Answer from the drawing. Dimensions are ordinates in mm from the lowest x, y and z of the part. Coordinates: 2 decimals unless noted, no trailing zeros. Loops run counter-clockwise (first coordinate to the right, second up) from the corner with the lowest first, then second, coordinate; pieces in that order, holes last. Notation, with made-up numbers: (-2.5, 9.25) - (51.5, 9.25) arc R14 ccw to (51.5, 15.25) - close; hole circle Ø7 at (43.25, 18). An arc over 180 degrees is marked (long way). Write each question's results on one line, items separated by ' | '. Start each with the question number.
1. Find the intervals of material crossed by line 1 along X through (y, z) = (54, 5); line 2 along Y through (x, z) = (8, 5.5); line 3 along Z through (x, y) = (8, 3.5), in increasing order. Write a range as [from, to].
2. Determine the mould class of the marked faces 1, 2 and 3 for opening direction Z: released by +Z, released by -Z, zero draft, split by the parting line, or undercut.
3. A cutting plane is placed at D-D on y = 4.5. Determine the outline of the cut face in (x, z).
4. This flat-tipped pin is pushed along its axis until it touches: P1, Ø4.5, axis at x = 8, z = 8, coming from the -Y side. Where does it stop, or does it pass through?
5. A cutting plane is placed at B-B on x = 8. Determine the outline of the cut face in (y, z).
6. A cutting plane is placed at A-A on y = 54. Determine the outline of the cut face in (x, z), then the cut area to 3 significant figures.
7. A cutting plane is placed at C-C on z = 10.5. Determine the outline of the cut face in (x, y), then the cut area to 3 significant figures.
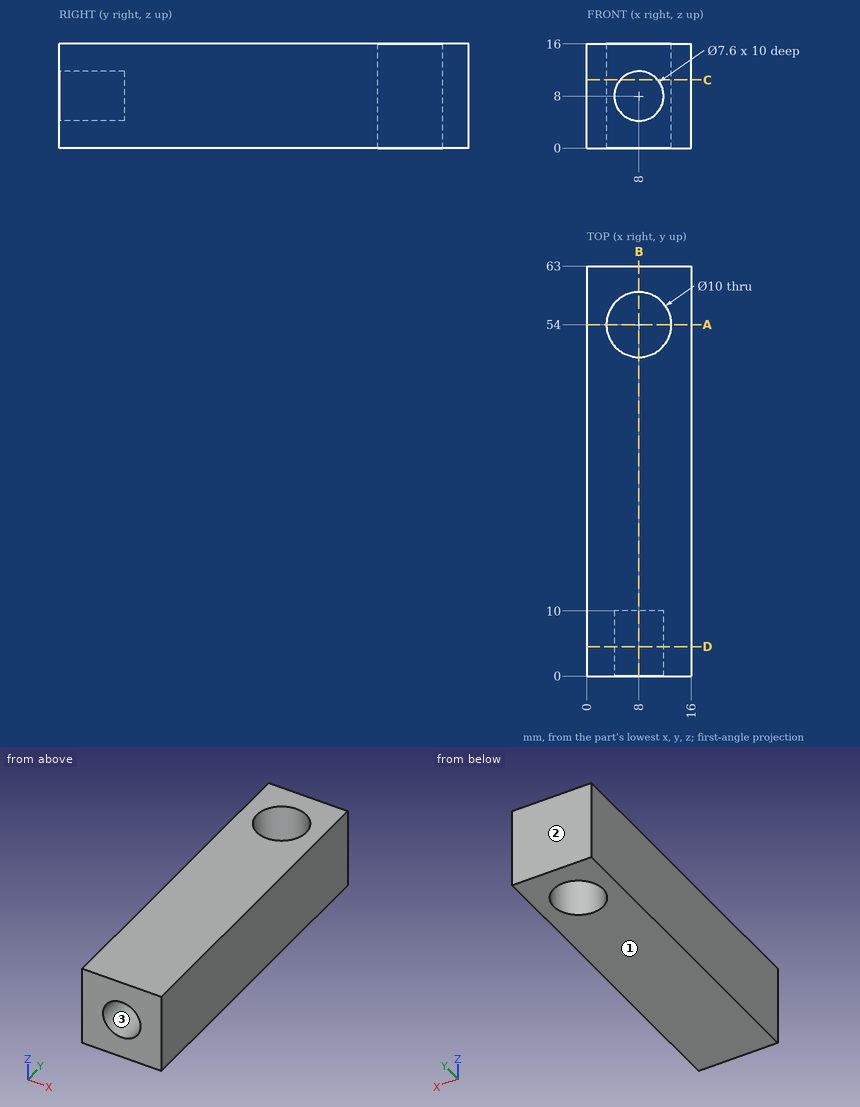
Values:
1) line 1: [0, 3], [13, 16] | line 2: [10, 49], [59, 63] | line 3: [0, 4.2], [11.8, 16]
2) face 1: released by -Z | face 2: zero draft | face 3: undercut
3) outline: (0, 0) - (16, 0) - (16, 16) - (0, 16) - close; hole circle Ø7.6 at (8, 8)
4) P1: y = 10
5) outline: (0, 0) - (49, 0) - (49, 16) - (0, 16) - (0, 11.8) - (10, 11.8) - (10, 4.2) - (0, 4.2) - close; (59, 0) - (63, 0) - (63, 16) - (59, 16) - close
6) outline: (0, 0) - (3, 0) - (3, 16) - (0, 16) - close; (13, 0) - (16, 0) - (16, 16) - (13, 16) - close | area: 96.0 mm^2
7) outline: (0, 0) - (5.14, 0) - (5.14, 10) - (10.86, 10) - (10.86, 0) - (16, 0) - (16, 63) - (0, 63) - close; hole circle Ø10 at (8, 54) | area: 872 mm^2
